Check sheet for the modelled part. Datum: model origin and axes. Units: mm. Give positions to 0.01 mm unless a question says otherwise; leave off trailing zeros. Order: outer loops, then holes, each group sorted by start corner. A loop starts at its lowest first (then second) coordinate and runs counter-clockwise, first axis right, second up. Notation, with made-up numbers: (63, -12) -> (93, -12) arc R14 ccw to (93, 7) -> close; hole circle Ø10 at (35, 88.25). An arc over 180 degrees is marked (long way). One line per question, with ' | ' between items.
```python
from build123d import *

# Parameters (mm, degrees)
SKETCH1_W           = 16
SKETCH1_H           = 24
SKETCH1_R           = 1.6
BOSS_EXTRUDE1_DEPTH = 3.175
FILLET1_R           = 2


with BuildPart() as part:
    # Sketch1 → Boss-Extrude1 (new body)
    with BuildSketch(Plane.XY):
        with Locations((0, -38)):
            Rectangle(SKETCH1_W, SKETCH1_H)
        with Locations((4, -30.85)):
            Circle(SKETCH1_R, mode=Mode.SUBTRACT)
        with Locations(Location((-4, -30.85, 0), (0, 0, 180))):
            Circle(SKETCH1_R, mode=Mode.SUBTRACT)
        with Locations((0, -46)):
            Circle(SKETCH1_R, mode=Mode.SUBTRACT)
    extrude(amount=BOSS_EXTRUDE1_DEPTH)

    # Fillet1
    fillet1_edges = [part.edges().sort_by_distance(p)[0] for p in [
        (8, -50, 1.5875),
        (-8, -50, 1.5875),
    ]]
    fillet(fillet1_edges, radius=FILLET1_R)


solid = part.part
```
Q1. Mould release check, pull along Y, two halves, no side actions. Record for faces 1 (the face through (-8, -37, 2)), 2 (the face through (0, -26, 2)), 3 (the face through (0.74, -47.42, 1.57)), 4 (the face through (0, -50, 2)): pulls with the +Y half, pulls with the -Y half, needs draft (parallel to the pull), parting line crosses it, or undercut.
Result sheet:
face 1: needs draft | face 2: pulls with the +Y half | face 3: undercut | face 4: pulls with the -Y half
Q2. Section check B-B (z = 1.3). Enter the section's corners in (x, y), and give its area (3 significant figures).
Result sheet:
outline: (-8, -48) arc R2 ccw to (-6, -50) -> (6, -50) arc R2 ccw to (8, -48) -> (8, -26) -> (-8, -26) -> close; hole circle Ø3.2 at (-4, -30.85); hole circle Ø3.2 at (0, -46); hole circle Ø3.2 at (4, -30.85) | area: 358 mm2
Q3. Thickness scan on line 1 (Y direction, x = 4, z = 0.5); line 2 (Y direction, x = 0, z = 1.5); line 3 (X direction, y = -31.75, z = 1.3). Record the ranges inside material, lowest first.
Result sheet:
line 1: y = -50 to -32.45, -29.25 to -26 | line 2: y = -50 to -47.6, -44.4 to -26 | line 3: x = -8 to -5.32, -2.68 to 2.68, 5.32 to 8
Q4. Section check D-D (x = -3). Enter the section's corners in (y, z) (3 decimals), and give its area (3 significant figures).
Result sheet:
outline: (-50, 0) -> (-32.099, 0) -> (-32.099, 3.175) -> (-50, 3.175) -> close; (-29.601, 0) -> (-26, 0) -> (-26, 3.175) -> (-29.601, 3.175) -> close | area: 68.3 mm2
Q5. Section check C-C (y = -32). Enter the section's corners in (x, z) (3 decimals).
Result sheet:
outline: (-8, 0) -> (-5.112, 0) -> (-5.112, 3.175) -> (-8, 3.175) -> close; (-2.888, 0) -> (2.888, 0) -> (2.888, 3.175) -> (-2.888, 3.175) -> close; (5.112, 0) -> (8, 0) -> (8, 3.175) -> (5.112, 3.175) -> close
Q6. Section check A-A (x = 4). Enter the section's corners in (y, z) (3 decimals), and give its area (3 significant figures).
Result sheet:
outline: (-50, 0) -> (-32.45, 0) -> (-32.45, 3.175) -> (-50, 3.175) -> close; (-29.25, 0) -> (-26, 0) -> (-26, 3.175) -> (-29.25, 3.175) -> close | area: 66.0 mm2
Q7. Depth check by flat-ended pin: pin 1 Ø2.5 at (x, y) = (-4, -30.85) entering from -Z. Enter the tip coordinate at first touch or a pass-through.
Result sheet:
pin 1: passes through
